Answer from the drawing. Dimensions are ordinates in mm from the lowest x, y and z of the part. Round coordinates to 2 decimals unless told otherwise and drop trailing zeros. Loops run counter-clockwise (first coordinate to the right, second up) from the corner with the lowest first, then second, coordinate; pieces in that order, holes last. Notation, with made-up numbers: (53.25, 37.5) -> (111.25, 37.5) arc R28 ccw to (111.25, 62.5) -> close; hole circle Ø11 at (-21, 66). An arc over 180 degrees is marked (long way). One line per question, with ' | ' between items.
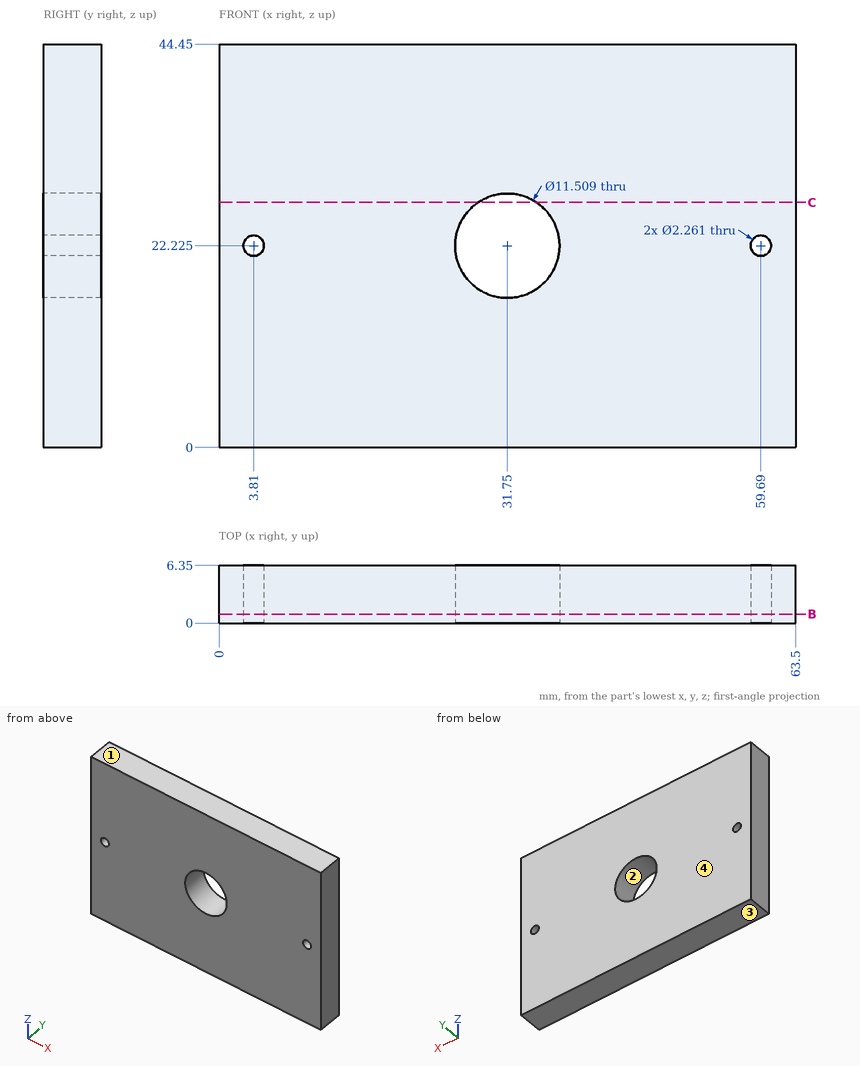
Q1. For a pull along Z with two mould halves and no side action, classify the marked faces 1, 2, 3 and 4 as pulls with the +Z half, pulls with the -Z half, needs draft (parallel to the pull), parting line crosses it, or undercut.
Numbers:
face 1: pulls with the +Z half | face 2: undercut | face 3: pulls with the -Z half | face 4: needs draft
Q2. A cutting plane is placed at B-B on y = 1. Give the number of separate pieces and of enclosed holes in the cut face, plus the area to 3 significant figures.
Numbers:
separate pieces: 1 | enclosed holes: 3 | area: 2,710 mm^2
Q3. A cutting plane is placed at C-C on z = 27. Give the vertices of the cut face in (x, y).
Numbers:
outline: (0, 0) -> (28.54, 0) -> (28.54, 6.35) -> (0, 6.35) -> close; (34.96, 0) -> (63.5, 0) -> (63.5, 6.35) -> (34.96, 6.35) -> close
Q4. Find the intervals of material crossed by line 1 (Z direction, x = 31.75, y = 4.25); line 2 (X direction, y = 3.5, z = 25); line 3 (X direction, y = 5, z = 19) (1 decimal), in increasing order. Write a range as from..to.
Numbers:
line 1: 0..16.47, 27.98..44.45 | line 2: 0..26.71, 36.79..63.5 | line 3: 0..27, 36.5..63.5
